Autodesk Inventor part; units mm, degrees
ref_plane "YZ Plane" through (0, 0, 0) normal (1, 0, 0) x (0, 1, 0)
ref_plane "XZ Plane" through (0, 0, 0) normal (0, 1, 0) x (-1, 0, 0)
ref_plane "XY Plane" through (0, 0, 0) normal (0, 0, 1) x (1, 0, 0)
sketch "Sketch1" plane through (0, 0, 0) normal (0, 0, 1) x (1, 0, 0)
  line L0 (-44.45, -6.35) -> (44.45, -6.35)
  line L1 (44.45, -6.35) -> (44.45, 6.35)
  line L2 (44.45, 6.35) -> (-44.45, 6.35)
  line L3 (-44.45, 6.35) -> (-44.45, -6.35)
  line L4 (-44.45, -6.35) -> (44.45, 6.35) construction
  line L5 (44.45, -6.35) -> (-44.45, 6.35) construction
  point P0 (0, 0)
  dimension "d0" = 88.9
  dimension "d1" = 12.7
extrude "Plate1" add sketch "Sketch1" along normal mid plane 6.35
fillet "Corner Round1" radius 6.35 4 edges at (-44.45, -6.35, 0) (-44.45, 6.35, 0) (44.45, 6.35, 0) (44.45, -6.35, 0)
sketch "Sketch4" plane through (0, 0, 3.175) normal (0, 0, 1) x (1, 0, 0)
  arc A0 (-38.1, 6.35) -> (-38.1, -6.35) centre (-38.1, 0) ccw construction
  arc A1 (38.1, -6.35) -> (38.1, 6.35) centre (38.1, 0) ccw construction
  point P0 (0, 0)
hole "Hole1" at (-38.1, 0, 3.175) at (38.1, 0, 3.175) direction (0, 0, -1) diameter 3.683 end through all
equation "\"d29\" = Thickness"
equation "\"d2\" = Thickness"
equation "\"BendRadius\" = Thickness"
equation "\"BendReliefWidth\" = Thickness"
equation "\"BendReliefDepth\" = 0.5 * Thickness"
equation "\"CornerReliefSize\" = 4 * Thickness"
equation "\"MinimumRemnant\" = 2 * Thickness"
equation "\"TransitionRadius\" = BendRadius"
equation "\"JacobiRadiusSize\" = BendRadius"
equation "\"GapSize\" = Thickness"
properties part number "MOUNT,STRAP,BATTERY" material "Aluminum 7075"
Source: CAD feature listing. Evaluate the final solid. Frame: model axes, mm. Round coordinates to 2 decimals unless told otherwise and drop trailing zeros. Loops run counter-clockwise (first coordinate to the right, second up) from the corner with the lowest first, then second, coordinate; pieces in that order, holes last.
Q1. Section D-D, the plane y = -4.25. Return loops of the section in (x, z) (3 decimals).
Q2. Section B-B, the plane y = 0.75. Return loops of the section in (x, z) (3 decimals).
Q3. Ray query, line 1 (X direction, y = 0, z = 0.5); line 2 (Y direction, x = 38.1, z = 1); line 3 (Y direction, x = -39.5, z = 0.25). Return the intervals inside material, ascending.
Q4. Section A-A, the plane z = 2. State how many separate pieces and enclosed holes the cut face has, plus the area to 3 significant figures.
Q5. Mould query, pull axis Y, two halves, no side actions, for faces 1 (the face through (-36.302, 0.399, -0.044)), 2 (the face through (36.274, 0.24, -0.044)), 3 (the face through (-1, -6.35, 0)), 4 (the face through (42.54, 4.54, -0.04)). Classes: pulls with the +Y half, pulls with the -Y half, needs draft (parallel to the pull), parting line crosses it, or undercut.
Q6. Section C-C, the plane y = 4. Return loops of the section in (x, z) (3 decimals).
Solutions:
1. outline: (-42.818, -3.175) - (42.818, -3.175) - (42.818, 3.175) - (-42.818, 3.175) - close
2. outline: (-44.406, -3.175) - (-39.782, -3.175) - (-39.782, 3.175) - (-44.406, 3.175) - close; (-36.418, -3.175) - (36.418, -3.175) - (36.418, 3.175) - (-36.418, 3.175) - close; (39.782, -3.175) - (44.406, -3.175) - (44.406, 3.175) - (39.782, 3.175) - close
3. line 1: x = -44.45 to -39.94, -36.26 to 36.26, 39.94 to 44.45
3. line 2: y = -6.35 to -1.84, 1.84 to 6.35
3. line 3: y = -6.19 to -1.2, 1.2 to 6.19
4. separate pieces: 1
4. enclosed holes: 2
4. area: 1,070 mm2
5. face 1: undercut
5. face 2: undercut
5. face 3: pulls with the -Y half
5. face 4: pulls with the +Y half
6. outline: (-43.032, -3.175) - (43.032, -3.175) - (43.032, 3.175) - (-43.032, 3.175) - close
